Design review of the part shown in the three views and the two pictorial views. Dimensions are in mm from the part's minimum x, y and z. Coordinates: 2 decimals unless noted, no trailing zeros. Write each loop counter-clockwise with the first axis right and the second up, starting at its lowest first coordinate (ties: lowest second). Pieces come first, ordered by that corner, then holes. Notation, with made-up numbers: (-32, 32.5) -> (4, 32.5) arc R35 cw to (4, 64.5) -> close; hole circle Ø6 at (-26.75, 76). An arc over 180 degrees is marked (long way). Answer in a Markdown table with one row per item. Add a question column.
Item 1: Draft analysis for pull direction X (two halves, no side actions). For the marked faces 1, 2 and 3, state which applies: released by +X, released by -X, zero draft, split by the parting line, or undercut.
Item 2: To check wall thickness, follow line 1 (X direction, y = 14, z = 7) (1 decimal); line 2 (Z direction, x = 171, y = 6) (1 decimal); line 3 (X direction, y = 3.75, z = 14.5) (1 decimal). State the ranges of each line that lie inside material, in increasing order.
Item 3: Take a section at A-A, the plane z = 19.75. Write out the cut boundary in (x, y).
Item 4: Take a section at C-C, the plane y = 5.75. Give the number of separate pieces and of enclosed holes in the cut face, and give its area (3 significant figures).
Item 5: Take a section at D-D, the plane z = 27.75. Write out the cut boundary in (x, y), and give its area (3 significant figures).
Item 6: Clearance check with flat-ended pins moving along their axes: P1, Ø4.5, axis at x = 98.5, y = 2.5, coming from the -Z side; P2, Ø0.6, axis at y = 14, z = 10.5, coming from the +X side; P3, Ø2, axis at y = 2, z = 18, coming from the -X side. State where each tip first meets the part, or that it passes through.
Item 7: Take a section at B-B, the plane x = 15.5. Write out the cut boundary in (y, z), and give its area (3 significant figures).
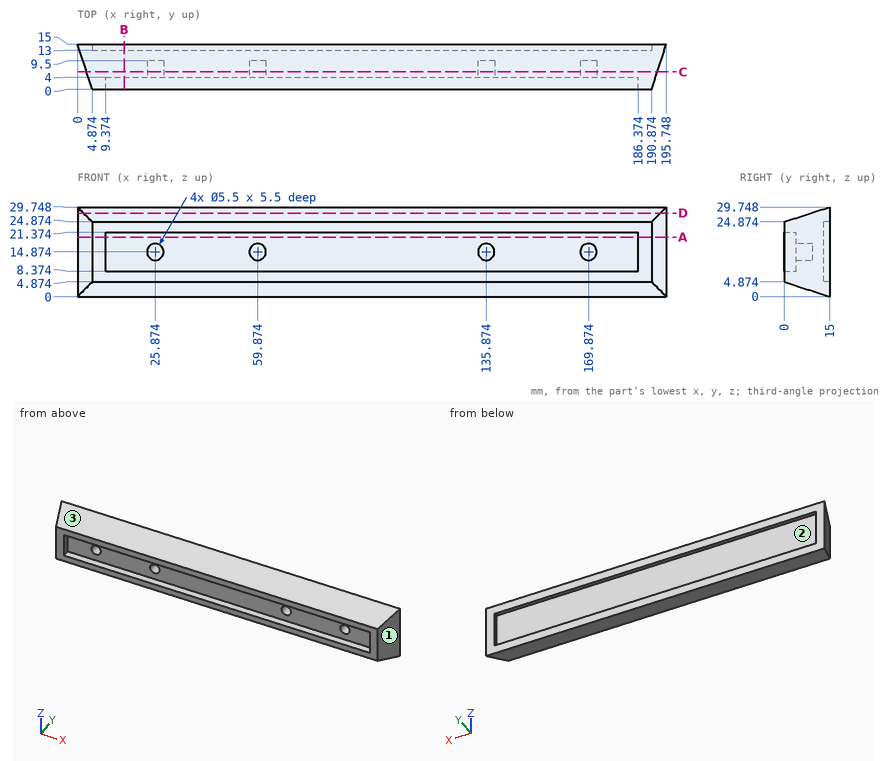
Answers:
| question | item | result |
|---|---|---|
| 1 | face 1 | released by +X |
| 1 | face 2 | undercut |
| 1 | face 3 | zero draft |
| 2 | line 1 | x = 0.3 to 4.9, 190.9 to 195.4 |
| 2 | line 2 | z = 2.9 to 12.4, 17.4 to 26.8 |
| 2 | line 3 | x = 3.7 to 9.4, 186.4 to 192.1 |
| 3 | outline | (0, 15) -> (4.87, 0) -> (9.37, 0) -> (9.37, 4) -> (186.37, 4) -> (186.37, 0) -> (190.87, 0) -> (195.75, 15) -> (190.87, 15) -> (190.87, 13) -> (4.87, 13) -> (4.87, 15) -> close |
| 4 | separate pieces | 1 |
| 4 | enclosed holes | 4 |
| 4 | area | 4,410 mm^2 |
| 5 | outline | (0, 15) -> (2, 8.85) -> (193.75, 8.85) -> (195.75, 15) -> close |
| 5 | area | 1,190 mm^2 |
| 6 | P1 | stops at z = 3.33 |
| 6 | P2 | stops at x = 195.52 |
| 6 | P3 | stops at x = 3.9 |
| 7 | outline | (0, 4.87) -> (15, 0) -> (15, 4.87) -> (13, 4.87) -> (13, 24.87) -> (15, 24.87) -> (15, 29.75) -> (0, 24.87) -> (0, 21.37) -> (4, 21.37) -> (4, 8.37) -> (0, 8.37) -> close |
| 7 | area | 281 mm^2 |
